```python
from build123d import *

# Parameters (mm, degrees)
SKETCH1_W           = 35
SKETCH1_H           = 1000
BOSS_EXTRUDE1_DEPTH = 7.5
SKETCH2_R           = 12.7
CUT_EXTRUDE1_DEPTH  = 8.5
LPATTERN1_COUNT     = 12
LPATTERN1_PITCH     = 55
FILLET1_R           = 10


with BuildPart() as part:
    # Sketch1 → Boss-Extrude1 (new body, symmetric)
    with BuildSketch(Plane.XY):
        Rectangle(SKETCH1_W, SKETCH1_H)
    extrude(amount=BOSS_EXTRUDE1_DEPTH, both=True)

    # Sketch2 → Cut-Extrude1 (cut, symmetric)
    with BuildSketch(Plane.XY):
        with Locations((0, -150)):
            Circle(SKETCH2_R)
    cut_extrude1 = extrude(amount=CUT_EXTRUDE1_DEPTH, both=True, mode=Mode.SUBTRACT)

    # LPattern1: Cut-Extrude1 ×12
    with Locations(*[(0, i * LPATTERN1_PITCH, 0) for i in range(1, LPATTERN1_COUNT)]):
        add(cut_extrude1, mode=Mode.SUBTRACT)

    # Fillet1
    fillet1_edges = [part.edges().sort_by_distance(p)[0] for p in [
        (-17.5, 500, 0),
        (17.5, 500, 0),
    ]]
    fillet(fillet1_edges, radius=FILLET1_R)


solid = part.part
```
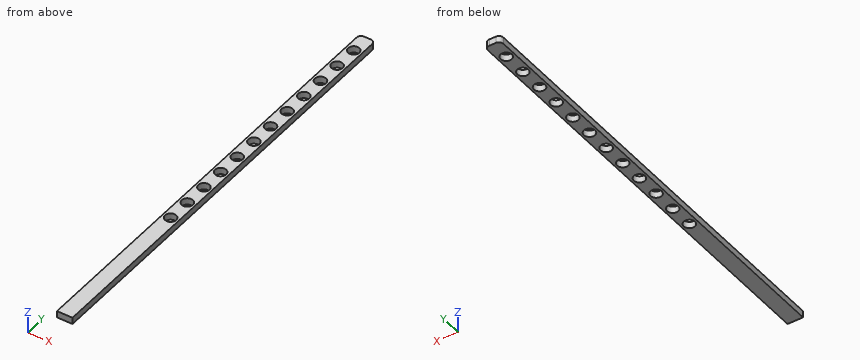
Geometry check sheet. Reference: the model listing, model coordinates, mm. Round coordinates to 2 decimals unless told otherwise and drop trailing zeros. Order: outer loops, then holes, each group sorted by start corner. A loop starts at its lowest first (then second) coordinate and runs counter-clockwise, first axis right, second up. Notation, with made-up numbers: (-30, 61) - (6, 61) arc R14 ccw to (6, 73) - close; hole circle Ø1 at (-9, -24). An arc over 180 degrees is marked (long way). Use a Markdown table: item, result. Add a question column.
(1) Sectioned sample at B-B, the plane z = -0.75. Count the separate pieces of the cut face and the enclosed holes in it, and give its area (3 significant figures).
(2) Sectioned sample at A-A, the plane y = 400. Enter the section's corners in (x, z), and give its area (3 significant figures).
(3) Depth check by flat-ended pin: pin 1 (20.5 mm diameter, centred on x = 0, y = -40, fed in from +Z). Enter the tip coordinate at first touch or a pass-through.
(4) Material ranges on line 1 along X through (y, z) = (123, 5); line 2 along X through (y, z) = (116.5, 3); line 3 along Y through (x, z) = (15, 5.75), recorded low to high. Write a range as [from, to].
Answers below:
| question | item | result |
|---|---|---|
| 1 | separate pieces | 1 |
| 1 | enclosed holes | 12 |
| 1 | area | 28,900 mm² |
| 2 | outline | (-17.5, -7.5) - (-12.7, -7.5) - (-12.7, 7.5) - (-17.5, 7.5) - close; (12.7, -7.5) - (17.5, -7.5) - (17.5, 7.5) - (12.7, 7.5) - close |
| 2 | area | 144 mm² |
| 3 | pin 1 | through |
| 4 | line 1 | [-17.5, -12.54], [12.54, 17.5] |
| 4 | line 2 | [-17.5, -9.44], [9.44, 17.5] |
| 4 | line 3 | [-500, 496.61] |
